Read the model definition and answer for the solid it produces. Units are mm, in the model's axes. Face numbers are marked on the shaded views. A direction names the side the tool comes from. Coordinates: 2 decimals unless noted, no trailing zeros. Order: outer loops, then holes, each group sorted by start corner. A loop starts at its lowest first (then second) coordinate and runs counter-clockwise, first axis right, second up. Notation, with made-up numbers: (77.25, -33.75) - (126.25, -33.75) arc R29 ccw to (126.25, 5.25) - close; hole circle Ø7 at (66, 55.25). An arc over 180 degrees is marked (long way). Use one line per item in the form item = value.
```python
from build123d import *

# Parameters (mm, degrees)
SKETCH2_W           = 155
SKETCH2_H           = 78
BOSS_EXTRUDE1_DEPTH = 21
BOSS_EXTRUDE2_DEPTH = 64
FILLET1_R           = 18
CUT_EXTRUDE1_DEPTH  = 22
SKETCH5_R           = 10.5
BOSS_EXTRUDE3_DEPTH = 21


with BuildPart() as part:
    # Sketch2 → Boss-Extrude1 (new body)
    with BuildSketch(Plane.XY):
        with Locations((77.5, 39)):
            Rectangle(SKETCH2_W, SKETCH2_H)
    extrude(amount=BOSS_EXTRUDE1_DEPTH)

    # Sketch3 → Boss-Extrude2 (add)
    with BuildSketch(Plane.XY.offset(21)):
        with BuildLine():
            Line((0, 0), (53.5, 0))
            ThreePointArc((53.5, 0), (77.5, 24), (101.5, 0))
            Line((101.5, 0), (155, 0))
            Line((155, 0), (155, 15))
            Line((155, 15), (105.5, 15))
            Line((105.5, 15), (105.5, 36))
            Line((105.5, 36), (49.5, 36))
            Line((49.5, 36), (49.5, 15))
            Line((49.5, 15), (0, 15))
            Line((0, 15), (0, 0))
        make_face()
    extrude(amount=BOSS_EXTRUDE2_DEPTH)

    # Fillet1
    fillet1_edges = [part.edges().sort_by_distance(p)[0] for p in [
        (0, 7.5, 85),
        (155, 7.5, 85),
    ]]
    fillet(fillet1_edges, radius=FILLET1_R)

    # Sketch4 → Cut-Extrude1 (cut, through all)
    with BuildSketch(Plane.XY.offset(21)):
        Polygon((0, 15), (56.725454791, 78), (0, 78), align=None)
        Polygon((155, 15), (98.274545209, 78), (155, 78), align=None)
    extrude(amount=-CUT_EXTRUDE1_DEPTH, mode=Mode.SUBTRACT)

    # Sketch5 → Boss-Extrude3 (add)
    with BuildSketch(Plane(origin=(0, 78, 0), x_dir=(1, 0, 0), z_dir=(0, 1, 0))):
        with BuildLine():
            Line((56.725454791, 0), (56.725454791, -35))
            ThreePointArc((56.725454791, -35), (77.5, -55.774545209), (98.274545209, -35))
            Line((98.274545209, -35), (98.274545209, 0))
            Line((98.274545209, 0), (56.725454791, 0))
        make_face()
        with Locations((77.5, -35)):
            Circle(SKETCH5_R, mode=Mode.SUBTRACT)
    extrude(amount=-BOSS_EXTRUDE3_DEPTH)


solid = part.part
```
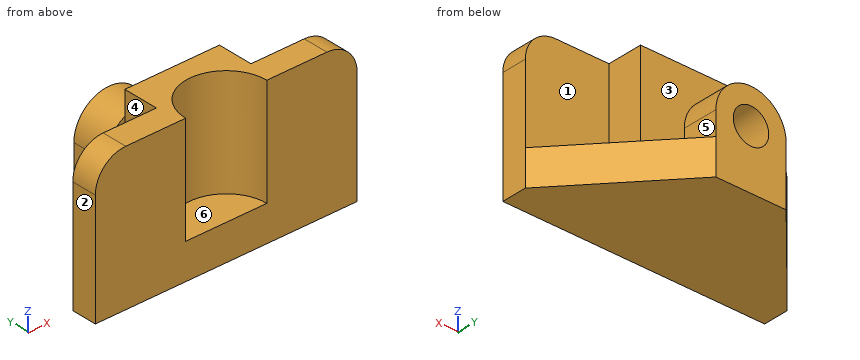
(1) Straight lines are drawn through the part: L1, parallel to X at y = 62, z = 35; L2, parallel to Z at x = 77.5, y = 69; L3, parallel to Y at x = 40, z = 53.5. For each, find the intervals that lie inside material, in ascending order.
Answer list:
L1 = 56.73 to 67, 88 to 98.27
L2 = 0 to 24.5, 45.5 to 55.77
L3 = 0 to 15
(2) Section A-A, the plane x = 77.5 is taken. Write down the section's boundary in (y, z), then the cut area to 3 significant figures.
Answer list:
outline = (0, 0) - (78, 0) - (78, 24.5) - (57, 24.5) - (57, 21) - (36, 21) - (36, 85) - (24, 85) - (24, 21) - (0, 21) - close; (57, 45.5) - (78, 45.5) - (78, 55.77) - (57, 55.77) - close
area = 2,700 mm2
(3) Which of the six approach directions +Z, -Z, +X, -X, +Y, -Y give full straight-line access (tool end or side, diameter ignored) to the marked faces 4, 5 and 6?
Answer list:
face_4 = +Z, -X, +Y
face_5 = +Z, +X, +Y
face_6 = +Z, -Y
(4) Given pin 1 Ø2 at (y, z) = (60, 34) entering from +X; pin 2 Ø7 at (x, y) = (71.5, 14.5) entering from +Z; pin 3 Ø17 at (x, z) = (77.5, 35) entering from -Y, each flat-ended and moving along its own axis, determine where each tip first touches the part or whether it passes through.
Answer list:
pin_1 = 98.27
pin_2 = 21
pin_3 = 22.44
(5) Section C-C, the plane y = 62.5 is taken. Write down the section's boundary in (x, z), then the cut area to 3 significant figures.
Answer list:
outline = (42.77, 0) - (112.23, 0) - (112.23, 21) - (98.27, 21) - (98.27, 35) arc R20.77 ccw to (56.73, 35) - (56.73, 21) - (42.77, 21) - close; hole circle Ø21 at (77.5, 35)
area = 2,370 mm2
(6) Section D-D, the plane z = 60 is taken. Write down the section's boundary in (x, y).
Answer list:
outline = (0, 0) - (53.5, 0) arc R24 cw to (101.5, 0) - (155, 0) - (155, 15) - (105.5, 15) - (105.5, 36) - (49.5, 36) - (49.5, 15) - (0, 15) - close
(7) The mould has two halves that part along Y. Classify the marked faces 1, 2 and 3: +Y half, -Y half, draft (parallel to the pull), parting line (faces both ways), or undercut.
Answer list:
face_1 = +Y half
face_2 = draft
face_3 = undercut
(8) Section B-B, the plane z = 30 is taken. Write down the section's boundary in (x, y).
Answer list:
outline = (0, 0) - (53.5, 0) arc R24 cw to (101.5, 0) - (155, 0) - (155, 15) - (105.5, 15) - (105.5, 36) - (49.5, 36) - (49.5, 15) - (0, 15) - close; (56.73, 57) - (68.27, 57) - (68.27, 78) - (56.73, 78) - close; (86.73, 57) - (98.27, 57) - (98.27, 78) - (86.73, 78) - close
